The listing builds one solid part. Answer for the finished solid, in the listing's coordinates (mm). Round coordinates to 2 decimals unless told otherwise and drop trailing zeros. Write each loop counter-clockwise with the first axis right and the second up, starting at its lowest first coordinate (ties: lowest second). Pieces come first, ordered by that corner, then holes.
Item 1: Find section B-B on x = 16. Give the vertices of the cut face in (y, z) (3 decimals), then the cut area to 3 significant figures.
Item 2: Find the intervals of material crossed by probe 1 along Y at (x, z) = (0, 0.5); probe 2 along X at (y, z) = (-31, 0.25); probe 3 along Y at (x, z) = (21.5, 1.25), in increasing order.
Item 3: Find section A-A on y = 0. Give the vertices of the cut face in (x, z) (3 decimals), then the cut area to 3 significant figures.
Item 4: Each of these flat-tipped pins is pushed along its axis until it touches: pin 1 (1.7 mm diameter, centred on x = -8, y = 0, fed in from +Z); pin 2 (3.5 mm diameter, centred on x = 0, y = -8, fed in from -Z); pin 3 (2.5 mm diameter, centred on y = -23, z = 1, fed in from -X); pin 4 (1.5 mm diameter, centred on y = 9.5, z = 1, fed in from +X). Where does it stop, or does it pass through?
Item 5: Find section D-D on y = -22. Give the vertices of the cut face in (x, z) (3 decimals), then the cut area to 3 significant figures.
Item 6: Find section C-C on x = -8. Give the vertices of the cut face in (y, z) (3 decimals), then the cut area to 3 significant figures.
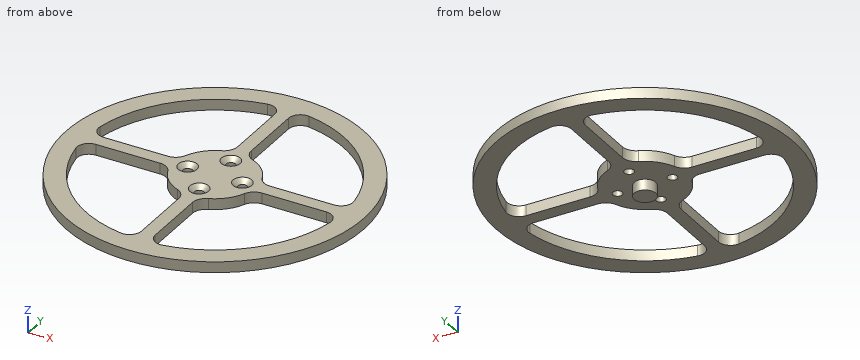
```python
from build123d import *

# Parameters (mm, degrees)
SKETCH1_R           = 43.5
SKETCH1_R_2         = 1.4
BOSS_EXTRUDE1_DEPTH = 3.175
FILLET1_R           = 4
FILLET2_R           = 3.5
SKETCH3_R           = 3.15
BOSS_EXTRUDE2_DEPTH = 3.175
CHAMFER1_SIZE       = 1.35


with BuildPart() as part:
    # Sketch1 → Boss-Extrude1 (new body)
    with BuildSketch(Plane.XY):
        Circle(SKETCH1_R)
        with Locations((0, 8)):
            Circle(SKETCH1_R_2, mode=Mode.SUBTRACT)
        with Locations((0, -8)):
            Circle(SKETCH1_R_2, mode=Mode.SUBTRACT)
        with Locations((8, 0)):
            Circle(SKETCH1_R_2, mode=Mode.SUBTRACT)
        with Locations((-8, 0)):
            Circle(SKETCH1_R_2, mode=Mode.SUBTRACT)
        with BuildLine():
            Line((-37.546770833, -2), (-11.882865816, -2))
            ThreePointArc((-11.882865816, -2), (-8.520636713, -8.520636713), (-2, -11.882865816))
            Line((-2, -11.882865816), (-2, -37.546770833))
            ThreePointArc((-2, -37.546770833), (-26.587214973, -26.587214973), (-37.546770833, -2))
        make_face(mode=Mode.SUBTRACT)
        with BuildLine():
            Line((-2, 37.546770833), (-2, 11.882865816))
            ThreePointArc((-2, 11.882865816), (-8.520636713, 8.520636713), (-11.882865816, 2))
            Line((-11.882865816, 2), (-37.546770833, 2))
            ThreePointArc((-37.546770833, 2), (-26.587214973, 26.587214973), (-2, 37.546770833))
        make_face(mode=Mode.SUBTRACT)
        with BuildLine():
            Line((2, 37.546770833), (2, 11.882865816))
            ThreePointArc((2, 11.882865816), (8.520636713, 8.520636713), (11.882865816, 2))
            Line((11.882865816, 2), (37.546770833, 2))
            ThreePointArc((37.546770833, 2), (26.587214973, 26.587214973), (2, 37.546770833))
        make_face(mode=Mode.SUBTRACT)
        with BuildLine():
            Line((11.882865816, -2), (37.546770833, -2))
            ThreePointArc((37.546770833, -2), (26.587214973, -26.587214973), (2, -37.546770833))
            Line((2, -37.546770833), (2, -11.882865816))
            ThreePointArc((2, -11.882865816), (8.520636713, -8.520636713), (11.882865816, -2))
        make_face(mode=Mode.SUBTRACT)
    extrude(amount=BOSS_EXTRUDE1_DEPTH)

    # Fillet1
    fillet1_edges = [part.edges().sort_by_distance(p)[0] for p in [
        (-11.882865816, 2, 1.5875),
        (-2, 11.882865816, 1.5875),
        (-2, -11.882865816, 1.5875),
        (-11.882865816, -2, 1.5875),
        (11.882865816, -2, 1.5875),
        (2, -11.882865816, 1.5875),
        (2, 11.882865816, 1.5875),
        (11.882865816, 2, 1.5875),
    ]]
    fillet(fillet1_edges, radius=FILLET1_R)

    # Fillet2
    fillet2_edges = [part.edges().sort_by_distance(p)[0] for p in [
        (-2, 37.546770833, 1.5875),
        (-37.546770833, 2, 1.5875),
        (-37.546770833, -2, 1.5875),
        (-2, -37.546770833, 1.5875),
        (2, -37.546770833, 1.5875),
        (37.546770833, -2, 1.5875),
        (37.546770833, 2, 1.5875),
        (2, 37.546770833, 1.5875),
    ]]
    fillet(fillet2_edges, radius=FILLET2_R)

    # Sketch3 → Boss-Extrude2 (add)
    with BuildSketch(Plane(origin=(0, 0, 0), x_dir=(-1, 0, 0), z_dir=(0, 0, -1))):
        with Locations(Location((0, 0, 0), (0, 0, 180))):
            Circle(SKETCH3_R)
    extrude(amount=BOSS_EXTRUDE2_DEPTH)

    # Chamfer1
    chamfer1_edges = [part.edges().sort_by_distance(p)[0] for p in [
        (6.6, 0, 3.175),
        (-9.4, 0, 3.175),
        (-1.4, 8, 3.175),
        (-1.4, -8, 3.175),
    ]]
    chamfer(chamfer1_edges, length=CHAMFER1_SIZE)


solid = part.part
```
Check values:
1. outline: (-40.451, 0) - (-34.026, 0) - (-34.026, 3.175) - (-40.451, 3.175) - close; (-2, 0) - (2, 0) - (2, 3.175) - (-2, 3.175) - close; (34.026, 0) - (40.451, 0) - (40.451, 3.175) - (34.026, 3.175) - close
1. area: 53.5 mm2
2. probe 1: y = -43.5 to -9.4, -6.6 to 6.6, 9.4 to 43.5
2. probe 2: x = -30.52 to -21.28, -2 to 2, 21.28 to 30.52
2. probe 3: y = -37.82 to -30.85, -2 to 2, 30.85 to 37.82
3. outline: (-43.5, 0) - (-9.4, 0) - (-9.4, 1.825) - (-10.75, 3.175) - (-43.5, 3.175) - close; (-6.6, 0) - (-3.15, 0) - (-3.15, -3.175) - (3.15, -3.175) - (3.15, 0) - (6.6, 0) - (6.6, 1.825) - (5.25, 3.175) - (-5.25, 3.175) - (-6.6, 1.825) - close; (9.4, 0) - (43.5, 0) - (43.5, 3.175) - (10.75, 3.175) - (9.4, 1.825) - close
3. area: 275 mm2
4. pin 1: passes through
4. pin 2: stops at z = 0
4. pin 3: stops at x = -37.67
4. pin 4: stops at x = 42.61
5. outline: (-37.527, 0) - (-30.492, 0) - (-30.492, 3.175) - (-37.527, 3.175) - close; (-2, 0) - (2, 0) - (2, 3.175) - (-2, 3.175) - close; (30.492, 0) - (37.527, 0) - (37.527, 3.175) - (30.492, 3.175) - close
5. area: 57.4 mm2
6. outline: (-42.758, 0) - (-36.739, 0) - (-36.739, 3.175) - (-42.758, 3.175) - close; (-9.011, 0) - (-1.4, 0) - (-1.4, 1.825) - (-2.75, 3.175) - (-9.011, 3.175) - close; (1.4, 0) - (9.011, 0) - (9.011, 3.175) - (2.75, 3.175) - (1.4, 1.825) - close; (36.739, 0) - (42.758, 0) - (42.758, 3.175) - (36.739, 3.175) - close
6. area: 84.7 mm2
